Geometry check sheet. Reference: the model listing, model coordinates, mm. A direction names the side the tool comes from. Round coordinates to 2 decimals unless told otherwise and drop trailing zeros. Write each loop counter-clockwise with the first axis right and the second up, starting at its lowest first coordinate (ties: lowest second). Pieces come first, ordered by that corner, then holes. Notation, with made-up numbers: M 83.25,56 L 133.25,56 A5 ccw 133.25,63 Z; hole C -7.5,-35 d4. An arc over 180 degrees is marked long. Put each result on its own line as item: value. Start each with the question number.
(1) Section check C-C on z = 5. Record the cut outline in (x, y).
(2) Section check B-B on y = 11.5. Record the cut outline in (x, z), then the cut area to 3 significant figures.
(3) Section check D-D on z = -78.83. Record the cut outline in (x, y).
(4) Tool access check on faces 4 (the flat face through (-75, 20.638, -44)), 5 (the flat face through (80, 7.938, 44)), 6 (the flat face through (-77, 11, -22.058)), 7 (the flat face through (-85.853, 11, -73)). Record the directions out of +Z, -Z, +X, -X, +Y, -Y that give a thin tool (end or side, any length) a straight path to the whole face; none if there is none.
(5) Material ranges on probe 1 along X at (y, z) = (0.85, 78.65); probe 2 along Z at (x, y) = (-77.5, 6.25); probe 3 along X at (y, z) = (6, 38), recorded low to high.
(6) Gauge pin test, flat ends, axial feed: pin 1 (10 mm diameter, centred on y = 18.5, z = 29, fed in from +X); pin 2 (2.5 mm diameter, centred on x = 79.92, z = 78.65, fed in from -Y); pin 3 (3 mm diameter, centred on x = -24, z = 10, fed in from +Y); pin 4 (16 mm diameter, centred on x = -78, z = -49, fed in from +Y). Record the tip position at first contact, or that the pin passes through.
(7) Mould release check, pull along Z, two halves, no side actions. Record for faces 1 (the flat face through (-58.4, 14, 33)), 2 (the cylindrical face through (41.7, 0.8, -54.1)), 3 (the flat face through (-74, 11, -82.227)): pulls with the +Z half, pulls with the -Z half, needs draft (parallel to the pull), parting line crosses it, or undercut.
(8) Section check A-A on z = 78.65. Record the cut outline in (x, y).
from build123d import *

# Parameters (mm, degrees)
SKETCH1_W                     = 170
SKETCH1_H                     = 170
BOSS_EXTRUDE1_DEPTH           = 1.5875
SKETCH2_W                     = 19.874317931
SKETCH2_H                     = 31.449470131
VGA_DEPTH                     = 19.05
SKETCH3_W                     = 19.655918832
SKETCH3_H                     = 22.058308912
HDMI_DEPTH                    = 19.05
SKETCH4_W                     = 28.391882757
SKETCH4_H                     = 17.471927851
USB_1_DEPTH                   = 25.4
SKETCH5_W                     = 27.955084562
SKETCH5_H                     = 20.092717029
ETH_USB_2_DEPTH               = 25.4
SKETCH6_W                     = 6.115174748
SKETCH6_H                     = 22.713506206
FRONT_USB_3_HEADER_DEPTH      = 6.35
SKETCH7_W                     = 11.356753103
SKETCH7_H                     = 48.921397982
ATX_DEPTH                     = 6.35
SKETCH8_W                     = 23.150304402
SKETCH8_H                     = 18.78232244
USB_MOUSE_DEPTH               = 19.05
SKETCH9_R                     = 2.015
LGA_1150_MOUNTING_HOLES_DEPTH = 126.64606768
MAIN_MOUNTING_HOLES_OUTLINE_R = 2.032
MAIN_MOUNTING_HOLES_DEPTH     = 1.5875


# Read off the part's stored shape, not the designer's step: Main Mounting holes
with BuildPart() as part:
    # Sketch1 → Boss-Extrude1 (new body)
    with BuildSketch(Plane(origin=(0, 0, 0), x_dir=(1, 0, 0), z_dir=(0, 1, 0))):
        Rectangle(SKETCH1_W, SKETCH1_H)
    extrude(amount=BOSS_EXTRUDE1_DEPTH)

    # Sketch2 → VGA (add)
    with BuildSketch(Plane(origin=(0, 1.5875, 0), x_dir=(1, 0, 0), z_dir=(0, 1, 0))):
        with Locations((-75.238489308, 43.35222098)):
            Rectangle(SKETCH2_W, SKETCH2_H)
    extrude(amount=VGA_DEPTH)

    # Sketch3 → HDMI (add)
    with BuildSketch(Plane(origin=(0, 1.5875, 0), x_dir=(1, 0, 0), z_dir=(0, 1, 0))):
        with Locations((-77.182705778, 11.029154456)):
            Rectangle(SKETCH3_W, SKETCH3_H)
    extrude(amount=HDMI_DEPTH)

    # Sketch4 → USB_1 (add)
    with BuildSketch(Plane(origin=(0, 1.5875, 0), x_dir=(1, 0, 0), z_dir=(0, 1, 0))):
        with Locations((-74.780315699, -11.029154456)):
            Rectangle(SKETCH4_W, SKETCH4_H)
    extrude(amount=USB_1_DEPTH)

    # Sketch5 → ETH_USB_2 (add)
    with BuildSketch(Plane(origin=(0, 1.5875, 0), x_dir=(1, 0, 0), z_dir=(0, 1, 0))):
        with Locations((-72.377925619, -33.087463367)):
            Rectangle(SKETCH5_W, SKETCH5_H)
    extrude(amount=ETH_USB_2_DEPTH)

    # Sketch6 → Front USB 3 Header (add)
    with BuildSketch(Plane(origin=(0, 1.5875, 0), x_dir=(1, 0, 0), z_dir=(0, 1, 0))):
        with Locations((80.064644879, -44.44421647)):
            Rectangle(SKETCH6_W, SKETCH6_H)
    extrude(amount=FRONT_USB_3_HEADER_DEPTH)

    # Sketch7 → ATX (add)
    with BuildSketch(Plane(origin=(0, 1.5875, 0), x_dir=(1, 0, 0), z_dir=(0, 1, 0))):
        with Locations((77.880653897, 45.099413765)):
            Rectangle(SKETCH7_W, SKETCH7_H)
    extrude(amount=ATX_DEPTH)

    # Sketch8 → USB_MOUSE (add)
    with BuildSketch(Plane(origin=(0, 1.5875, 0), x_dir=(1, 0, 0), z_dir=(0, 1, 0))):
        with Locations((-74.278230021, 72.836099228)):
            Rectangle(SKETCH8_W, SKETCH8_H)
    extrude(amount=USB_MOUSE_DEPTH)

    # Sketch9 → LGA 1150 Mounting holes (cut, through all)
    with BuildSketch(Plane(origin=(0, 1.5875, 0), x_dir=(1, 0, 0), z_dir=(0, 1, 0))):
        with Locations(Location((-33.43759867, 52.088184905, 0), (0, 0, 270))):
            Circle(SKETCH9_R)
        with Locations(Location((41.56240133, 52.088184905, 0), (0, 0, 270))):
            Circle(SKETCH9_R)
        with Locations(Location((41.56240133, -22.911815095, 0), (0, 0, 270))):
            Circle(SKETCH9_R)
        with Locations(Location((-33.43759867, -22.911815095, 0), (0, 0, 270))):
            Circle(SKETCH9_R)
    extrude(amount=-LGA_1150_MOUNTING_HOLES_DEPTH, mode=Mode.SUBTRACT)

    # Main Mounting holes outline → Main Mounting holes (cut)
    with BuildSketch(Plane(origin=(0, 0, 0), x_dir=(1, 0, 0), z_dir=(0, 1, 0))):
        with Locations((79.924351727, 78.83)):
            Circle(MAIN_MOUNTING_HOLES_OUTLINE_R)
        with Locations((79.924351727, -78.65)):
            Circle(MAIN_MOUNTING_HOLES_OUTLINE_R)
        with Locations((-75.015648273, -78.65)):
            Circle(MAIN_MOUNTING_HOLES_OUTLINE_R)
        with Locations((-52.155648273, 78.83)):
            Circle(MAIN_MOUNTING_HOLES_OUTLINE_R)
    extrude(amount=MAIN_MOUNTING_HOLES_DEPTH, mode=Mode.SUBTRACT)


solid = part.part
Answers follow:
1. outline: M -88.98,1.59 L -85,1.59 L -85,0 L 85,0 L 85,1.59 L -60.58,1.59 L -60.58,26.99 L -88.98,26.99 Z
2. outline: M -88.98,2.29 L -60.58,2.29 L -60.58,19.77 L -88.98,19.77 Z; M -87.01,-22.06 L -67.35,-22.06 L -67.35,0 L -87.01,0 Z; M -86.36,23.04 L -58.4,23.04 L -58.4,43.13 L -86.36,43.13 Z; M -85.85,-82.23 L -62.7,-82.23 L -62.7,-63.44 L -85.85,-63.44 Z; M -85.18,-59.08 L -65.3,-59.08 L -65.3,-27.63 L -85.18,-27.63 Z
2. area: 2,550 mm^2
3. outline: M -85.85,1.59 L -85,1.59 L -85,0 L -54.19,0 L -54.19,1.59 L -62.7,1.59 L -62.7,20.64 L -85.85,20.64 Z; M -50.12,0 L 77.89,0 L 77.89,1.59 L -50.12,1.59 Z; M 81.96,0 L 85,0 L 85,1.59 L 81.96,1.59 Z
4. face 4: -Z, +X, -X, +Y
4. face 5: +Z, -Z, +X, +Y
4. face 6: -X, +Y
4. face 7: -Z, -X, +Y, -Y
5. probe 1: x = -85 to -77.05, -72.98 to 77.89, 81.96 to 85
5. probe 2: z = -82.23 to -63.44, -59.08 to -27.63, -22.06 to 0, 2.29 to 19.77, 23.04 to 43.13
5. probe 3: x = -86.36 to -58.4, 77.01 to 83.12
6. pin 1: stops at x = -58.4
6. pin 2: passes through
6. pin 3: stops at y = 1.59
6. pin 4: stops at y = 20.64
7. face 1: needs draft
7. face 2: undercut
7. face 3: pulls with the -Z half
8. outline: M -85,0 L -77.05,0 L -77.05,1.59 L -85,1.59 Z; M -72.98,0 L 77.89,0 L 77.89,1.59 L -72.98,1.59 Z; M 81.96,0 L 85,0 L 85,1.59 L 81.96,1.59 Z
